Model file for the job. Use its own axes, mm. Face numbers are marked on the shaded views. Round coordinates to 2 decimals unless told otherwise and drop trailing zeros. Loops run counter-clockwise (first coordinate to the right, second up) from the corner with the lowest first, then second, coordinate; pieces in that order, holes last. Notation, with made-up numbers: M 43.5,52.25 L 88.5,52.25 A18 ccw 88.5,58.25 Z; hole C -16.5,-15.75 d3. An arc over 180 degrees is marked long. Answer in a Markdown table with one row per item.
Solid Edge part; units mm, degrees
sketch "Sketch1" plane through (0, 85, 0) normal (0, 1, 0) x (-1, 0, 0)
  line L0 (175, 0) -> (145, -50)
  line L1 (145, -50) -> (125, -50)
  line L2 (125, -50) -> (95, 0)
  line L3 (95, 0) -> (175, 0)
  circle A0 centre (119.7267, -14) radius 7.5
  circle A1 centre (133.2754, -20.2001) radius 1.5
  circle A2 centre (135, -35) radius 1.5
extrude "Extrusionsausprägung_1" add sketch "Sketch1" against normal blind 20
properties material "(None)"
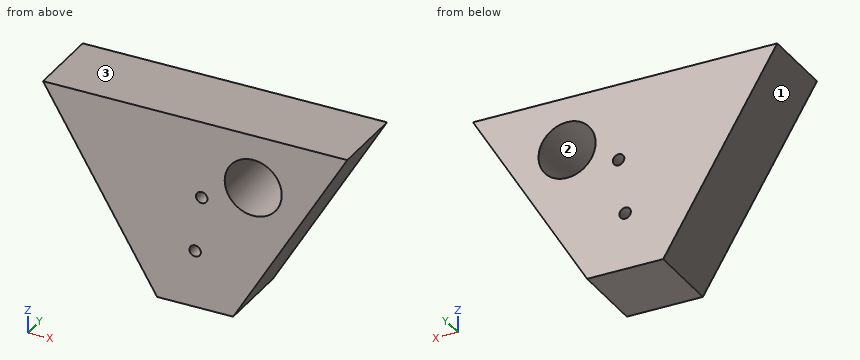
1. Saw through at C-C (y = 73). Write the cut outline in (x, z).
Verdict:
| item | result |
|---|---|
| outline | M -175,0 L -145,-50 L -125,-50 L -95,0 Z; hole C -135,-35 d3; hole C -133.28,-20.2 d3; hole C -119.73,-14 d15 |
2. Wall check: probe 1 along Z at (x, y) = (-135, 70.5); probe 2 along X at (y, z) = (70, -20); probe 3 along X at (y, z) = (75.5, -16.5). Give the ranges that are in metal, low to high.
Verdict:
| item | result |
|---|---|
| probe 1 | z = -50 to -36.5, -33.5 to 0 |
| probe 2 | x = -163 to -134.76, -131.79 to -124.23, -115.23 to -107 |
| probe 3 | x = -165.1 to -126.8, -112.66 to -104.9 |
3. Pin check, flat tips, straight feed: pin 1 (2 mm diameter, centred on y = 78, z = -31, fed in from +X); pin 2 (1 mm diameter, centred on y = 67, z = -19, fed in from -X); pin 3 (10 mm diameter, centred on y = 80.5, z = -26, fed in from +X). Stop position of each tip, or through.
Verdict:
| item | result |
|---|---|
| pin 1 | stops at x = -113 |
| pin 2 | stops at x = -163.9 |
| pin 3 | stops at x = -107.6 |
4. Saw through at B-B (x = -121). Write the cut outline in (y, z).
Verdict:
| item | result |
|---|---|
| outline | M 65,-43.33 L 85,-43.33 L 85,-21.39 L 65,-21.39 Z; M 65,-6.61 L 85,-6.61 L 85,0 L 65,0 Z |
5. Mould opens along X. For the marked faces 1, 2 and 3 say: +X half, -X half, draft (parallel to the pull), parting line (faces both ways), or undercut.
Verdict:
| item | result |
|---|---|
| face 1 | -X half |
| face 2 | undercut |
| face 3 | draft |
6. Saw through at D-D (z = -22.5). Write the cut outline in (x, y).
Verdict:
| item | result |
|---|---|
| outline | M -161.5,65 L -108.5,65 L -108.5,85 L -161.5,85 Z |
7. Saw through at A-A (z = -35). Write the cut outline in (x, y).
Verdict:
| item | result |
|---|---|
| outline | M -154,65 L -136.5,65 L -136.5,85 L -154,85 Z; M -133.5,65 L -116,65 L -116,85 L -133.5,85 Z |
